Here's the drawing with two shaded views (mm, measured from the low corner). I have some questions. A direction names the side the tool comes from. Give positions to 0.01 mm unless a question says otherwise; leave off trailing zeros. Write each loop counter-clockwise with the first axis right and the second up, starting at its lowest first coordinate (ties: lowest second). Pieces come first, ordered by that corner, then holes. Notation, with made-up numbers: (-16, 72) -> (10, 72) arc R20 cw to (10, 98) -> close; hole circle Ø10 at (12.5, -6.5). An arc over 180 degrees is marked (long way). One line per item, written item: value.
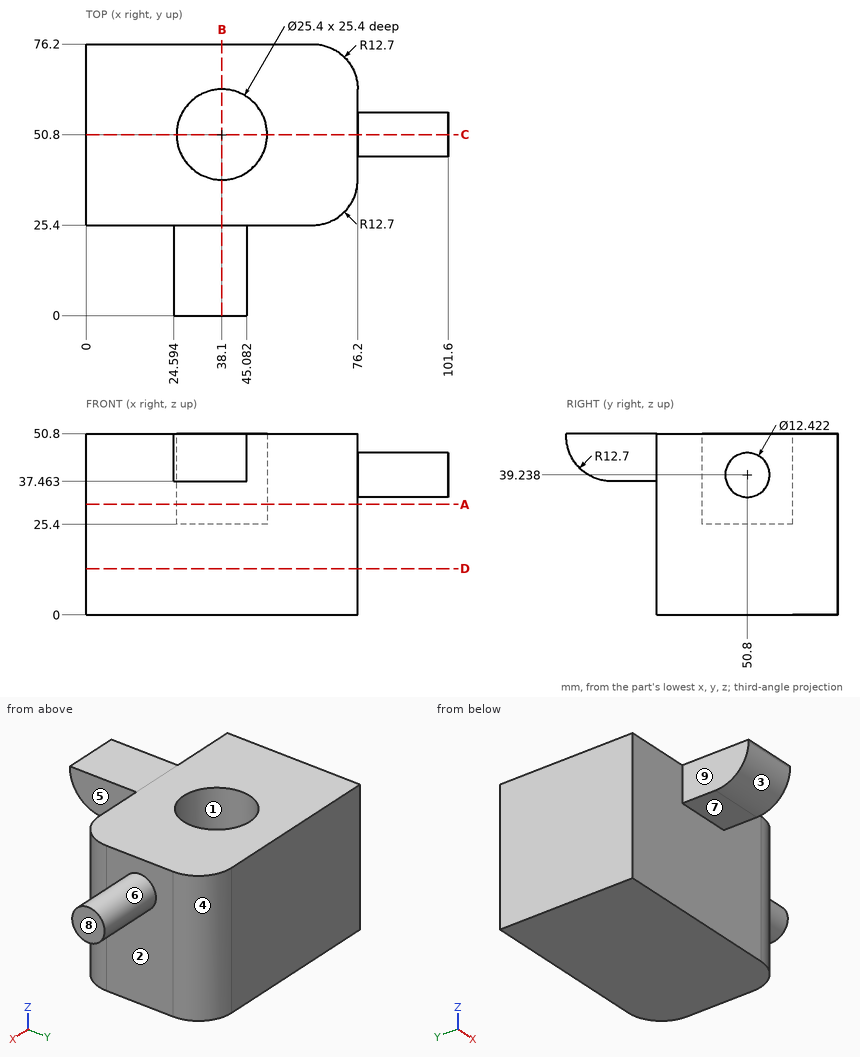
1) For the marked faces 5, 6, 7, 8 and 9, which set-ups out of +Z, -Z, +X, -X, +Y, -Y let a thin tool reach every point of the face, with its end or its side?
Answer list:
face 5: +Z, -Z, +X, -Y
face 6: +X
face 7: -Z, +X, -X, -Y
face 8: +Z, -Z, +X, +Y, -Y
face 9: +Z, -Z, -X, -Y
2) If we section it at D-D (z = 13): Write out the boundary of the cut face in (x, y), and give its area (3 significant figures).
Answer list:
outline: (0, 25.4) -> (63.5, 25.4) arc R12.7 ccw to (76.2, 38.1) -> (76.2, 63.5) arc R12.7 ccw to (63.5, 76.2) -> (0, 76.2) -> close
area: 3,800 mm^2
3) If we section it at B-B (x = 38.1): Write out the boundary of the cut face in (y, z), and give its area (3 significant figures).
Answer list:
outline: (0, 50.16) arc R12.7 ccw to (12.7, 37.46) -> (25.4, 37.46) -> (25.4, 0) -> (76.2, 0) -> (76.2, 50.8) -> (63.5, 50.8) -> (63.5, 25.4) -> (38.1, 25.4) -> (38.1, 50.8) -> (0, 50.8) -> close
area: 2,240 mm^2
4) If we section it at C-C (y = 50.8): Write out the boundary of the cut face in (x, z), and give its area (3 significant figures).
Answer list:
outline: (0, 0) -> (76.2, 0) -> (76.2, 33.03) -> (101.6, 33.03) -> (101.6, 45.45) -> (76.2, 45.45) -> (76.2, 50.8) -> (50.8, 50.8) -> (50.8, 25.4) -> (25.4, 25.4) -> (25.4, 50.8) -> (0, 50.8) -> close
area: 3,540 mm^2
5) If we section it at A-A (z = 31): Write out the boundary of the cut face in (x, y).
Answer list:
outline: (0, 25.4) -> (63.5, 25.4) arc R12.7 ccw to (76.2, 38.1) -> (76.2, 63.5) arc R12.7 ccw to (63.5, 76.2) -> (0, 76.2) -> close; hole circle Ø25.4 at (38.1, 50.8)
6) We'd pull the mould along Y, two halves only. Please class the marked faces 1, 2, 3 and 4: released by +Y, released by -Y, zero draft, split by the parting line, or undercut.
Answer list:
face 1: undercut
face 2: zero draft
face 3: released by -Y
face 4: released by +Y
7) Will these pins go through, and if not, where does the flat tip stop? pin 1 (2 mm diameter, centred on y = 60, z = 13, fed in from +X); pin 2 (12 mm diameter, centred on y = 19.5, z = 8, fed in from -X); pin 3 (15 mm diameter, centred on x = 47.5, z = 28, fed in from -Y); pin 4 (10 mm diameter, centred on x = 31, y = 18.5, fed in from -Z).
Answer list:
pin 1: stops at x = 76.2
pin 2: stops at x = 0
pin 3: stops at y = 25.4
pin 4: stops at z = 37.46
8) I need wall thicknesses on L1, parallel to X at y = 51, z = 37; L2, parallel to Y at x = 38.1, z = 44.25; L3, parallel to Y at x = 38.5, z = 35. Which ranges of each line are inside material? Lowest first, please.
Answer list:
L1: x = 0 to 25.4, 50.8 to 101.6
L2: y = 1.46 to 38.1, 63.5 to 76.2
L3: y = 25.4 to 38.11, 63.49 to 76.2
